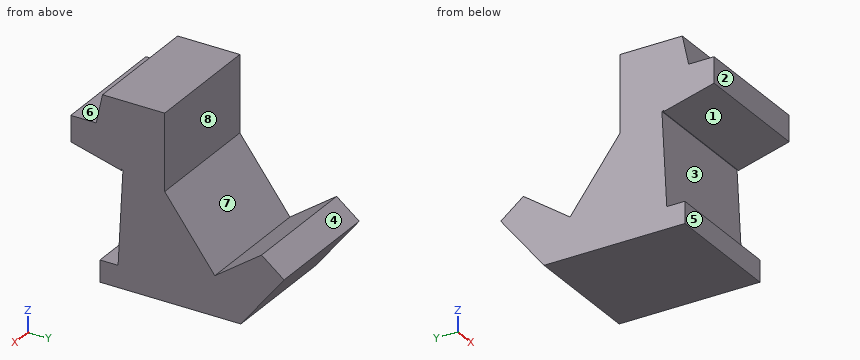
```python
from build123d import *

# Parameters (mm, degrees)
F0_W     = 88.9
F0_H     = 76.2
F1_DEPTH = 50.8
F4_DEPTH = 50.8
F7_DEPTH = 50.8


with BuildPart() as f1:
    # F0 (on Right) → F1 (new body)
    with BuildSketch(Plane.YZ):
        with Locations((44.45, 38.1)):
            Rectangle(F0_W, F0_H)
    extrude(amount=F1_DEPTH)

    # F2 (on face) → F4 (cut)
    with BuildSketch(Plane.YZ.offset(50.8)):
        Polygon((0, 76.2), (0, 64.015649), (10.592989, 64.015649), (13.236613, 76.2), align=None)
        Polygon((88.9, 76.2), (39.144106, 76.2), (39.144106, 44.45285), (60.028717, 16.43046), (79.499279, 30.397216), (88.9, 23.039514), align=None)
        Polygon((88.9, 23.039514), (70.867568, 0), (88.9, 0), align=None)
    extrude(amount=-F4_DEPTH, mode=Mode.SUBTRACT)

    # F6 (on face) → F7 (cut)
    with BuildSketch(Plane.YZ.offset(50.8)):
        Polygon((21.15212, 47.791194), (0, 53.31191), (0, 0), (12.17937, 0), (12.17937, 8.996861), (19.713309, 8.996861), (21.741677, 48.115388), (20.793015, 48.34297), align=None)
    extrude(amount=-F7_DEPTH, mode=Mode.SUBTRACT)


solid = f1.part
```
Source: CAD feature listing. Evaluate the final solid. Frame: model axes, mm. Face numbers are marked on the shaded views. A direction names the side the tool comes from. Give positions to 0.01 mm unless a question says otherwise; leave off trailing zeros. Loops run counter-clockwise (first coordinate to the right, second up) from the corner with the lowest first, then second, coordinate; pieces in that order, holes last. Notation, with made-up numbers: (26, 33) - (80, 33) arc R20 ccw to (80, 63) - close; hole circle Ø9 at (60.5, 49.25). An arc over 180 degrees is marked (long way). Use CSV: the item, a comma, the result in double quotes.
1) Cut plane C-C (x = 10). Output: boundary loops of the cut face in (y, z), and give its area (3 significant figures).
Worked out:
outline,"(0, 53.31) - (21.15, 47.79) - (20.79, 48.34) - (21.74, 48.12) - (19.71, 9) - (12.18, 9) - (12.18, 0) - (70.87, 0) - (88.9, 23.04) - (79.5, 30.4) - (60.03, 16.43) - (39.14, 44.45) - (39.14, 76.2) - (13.24, 76.2) - (10.59, 64.02) - (0, 64.02) - close"
area,"3,000 mm^2"
2) Pin query (flat end, axial travel): P1, Ø1.5, axis at x = 11, z = 25.5, coming from the -Y side; P2, Ø9.5, axis at x = 34.5, z = 60.5, coming from the +Y side; P3, Ø4, axis at x = 31.5, y = 70, coming from the -Z side; P4, Ø5.5, axis at x = 22, y = 5.5, coming from the +Z side. Return the tip coordinate at first contact, or that it passes through.
Worked out:
P1,"stops at y = 20.53"
P2,"stops at y = 39.14"
P3,"stops at z = 0"
P4,"stops at z = 64.02"
3) Cut plane D-D (z = 5.5). Output: boundary loops of the cut face in (x, y), and give its area (3 significant figures).
Worked out:
outline,"(0, 12.18) - (50.8, 12.18) - (50.8, 75.17) - (0, 75.17) - close"
area,"3,200 mm^2"
4) Set-up query: the marked faces 5, 6, 7 and 8. Return all of +Z, -Z, +X, -X, +Y, -Y with unobstructed straight access to the full face (end or side cutting, diameter ignored); none if empty.
Worked out:
face 5,"-Z, +X, -X, -Y"
face 6,"+Z, +X, -X, -Y"
face 7,"+Z, +X, -X"
face 8,"+Z, +X, -X, +Y"
5) Cut plane A-A (y = 16). Output: boundary loops of the cut face in (x, z), and give its area (3 significant figures).
Worked out:
outline,"(0, 0) - (50.8, 0) - (50.8, 9) - (0, 9) - close; (0, 49.14) - (50.8, 49.14) - (50.8, 76.2) - (0, 76.2) - close"
area,"1,830 mm^2"
6) Cut plane B-B (z = 25). Output: boundary loops of the cut face in (x, y).
Worked out:
outline,"(0, 20.54) - (50.8, 20.54) - (50.8, 53.64) - (0, 53.64) - close; (0, 71.98) - (50.8, 71.98) - (50.8, 86.4) - (0, 86.4) - close"
7) Line query: line 1 (Y direction, x = 44.5, z = 62); line 2 (Z direction, x = 33, y = 17); line 3 (Y direction, x = 26.5, z = 28.5). Output: solid intervals per line, ascending.
Worked out:
line 1,"y = 0 to 39.14"
line 2,"z = 0 to 9, 48.87 to 76.2"
line 3,"y = 20.72 to 51.03, 76.85 to 81.92"
8) Mould query, pull axis Z, two halves, no side actions, for the marked faces 1, 2, 3 and 4. Classes: +Z half, -Z half, draft (parallel to the pull), parting line (faces both ways), or undercut.
Worked out:
face 1,"undercut"
face 2,"draft"
face 3,"undercut"
face 4,"+Z half"
